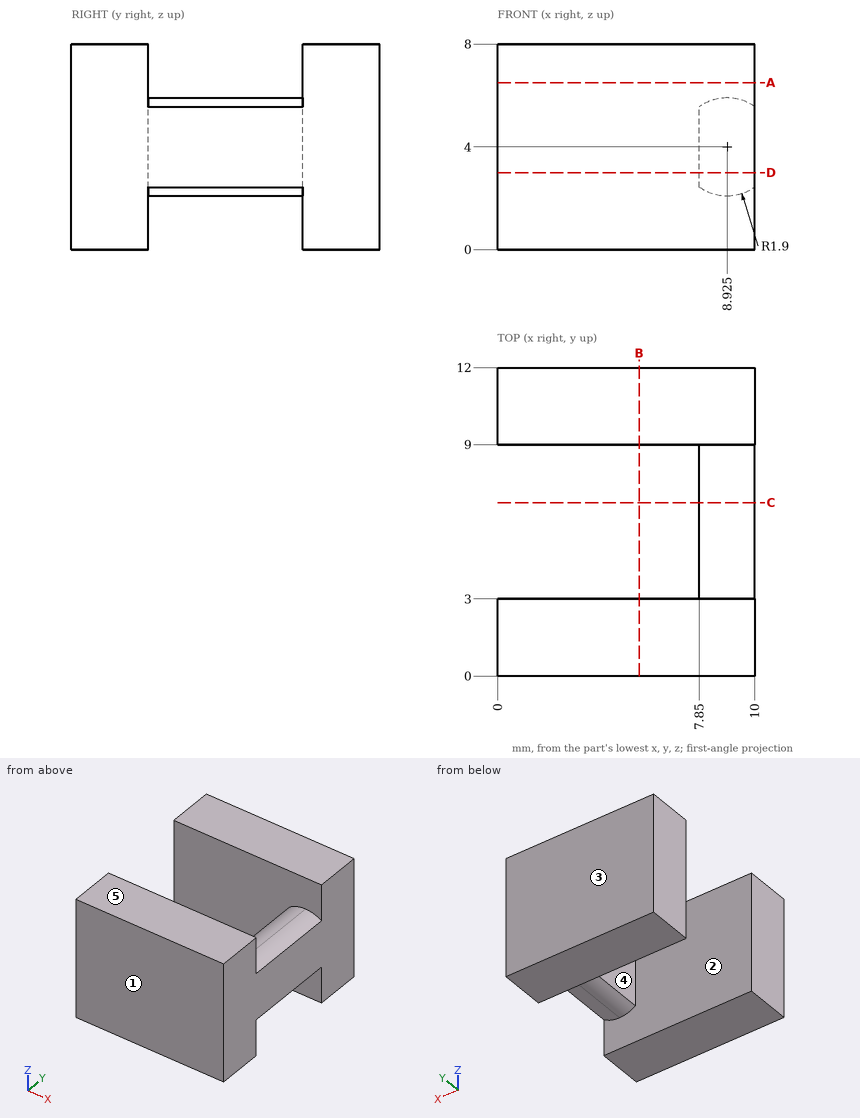
Could you check a few things on this drawing? It's one solid part, dimensions in mm from its lowest x, y, z. A direction names the side the tool comes from. Coordinates: 2 decimals unless noted, no trailing zeros. Order: outer loops, then holes, each group sorted by start corner. A loop starts at its lowest first (then second) coordinate and runs counter-clockwise, first axis right, second up. Notation, with made-up numbers: (-34.5, -0.5) - (-27.5, -0.5) arc R19 cw to (-27.5, 26.5) - close; hole circle Ø3 at (82.5, 50.25). An arc over 180 degrees is marked (long way). One line per question, with ' | ' between items.
(1) If I drill on L1, parallel to Y at x = 4, z = 4; L2, parallel to X at y = 5.5, z = 4.5, over which ranges is the centre line in solid material (lowest first)?
Report:
L1: y = 0 to 3, 9 to 12 | L2: x = 7.85 to 10
(2) Will this pin go through, and if not, where does the flat tip stop? pin 1 (0.9 mm diameter, centred on y = 5, z = 4, fed in from -X).
Report:
pin 1: stops at x = 7.85
(3) Suppose I cut it at A-A on z = 6.5. List the corners of the cut face in (x, y) for me.
Report:
outline: (0, 0) - (10, 0) - (10, 3) - (0, 3) - close; (0, 9) - (10, 9) - (10, 12) - (0, 12) - close
(4) If we mould it in two halves opening along Y, with no side actions, what happens to the marked faces 1, 2 and 3? For each: pulls with the +Y half, pulls with the -Y half, needs draft (parallel to the pull), parting line crosses it, or undercut.
Report:
face 1: pulls with the -Y half | face 2: undercut | face 3: pulls with the +Y half
(5) For the marked faces 4 and 5, which set-ups out of +Z, -Z, +X, -X, +Y, -Y let a thin tool reach every point of the face, with its end or its side?
Report:
face 4: +Z, -Z, -X | face 5: +Z, +X, -X, +Y, -Y
(6) Suppose I cut it at C-C on y = 6.75. List the corners of the cut face in (x, z) for me (3 decimals).
Report:
outline: (7.85, 2.433) arc R1.9 ccw to (10, 2.433) - (10, 5.567) arc R1.9 ccw to (7.85, 5.567) - close
(7) Suppose I cut it at D-D on z = 3. List the corners of the cut face in (x, y) for me.
Report:
outline: (0, 0) - (10, 0) - (10, 12) - (0, 12) - (0, 9) - (7.85, 9) - (7.85, 3) - (0, 3) - close
(8) Suppose I cut it at B-B on x = 5.5. List the corners of the cut face in (y, z) for me, and give its area (3 significant figures).
Report:
outline: (0, 0) - (3, 0) - (3, 8) - (0, 8) - close; (9, 0) - (12, 0) - (12, 8) - (9, 8) - close | area: 48.0 mm2
